Part model, mm, in its own coordinate system. Give positions to 0.01 mm unless a question says otherwise; leave off trailing zeros. Loops run counter-clockwise (first coordinate to the right, second up) from the corner with the lowest first, then second, coordinate; pieces in that order, holes last. Notation, with made-up numbers: (6, 71.5) -> (11, 71.5) arc R21 cw to (11, 93.5) -> close; hole circle Ø3 at (19, 34.25). An arc over 180 degrees is marked (long way). Write item = value, one per line.
from build123d import *

# Parameters (mm, degrees)
CYLINDER_R        = 0.34
CYLINDER_DEPTH    = 12.5
CYLINDER002_R     = 0.24
CYLINDER002_DEPTH = 2.65


with BuildPart() as cone:
    # Cone → Cone (revolve)
    with BuildSketch(Plane(origin=(0, 0, -3.55), x_dir=(1, 0, 0), z_dir=(0, -1, 0))):
        Polygon((0, 0), (0.24, 0.9), (0, 0.9), align=None)
    revolve(axis=Axis((0, 0, -3.55), (0, 0, 1)))


with BuildPart() as body:
    # Cylinder → Cylinder (new body)
    with BuildSketch(Plane.XY):
        Circle(CYLINDER_R)
    extrude(amount=CYLINDER_DEPTH)


with BuildPart() as pin:
    # Cylinder002 → Cylinder002 (new body)
    with BuildSketch(Plane.XY.offset(-2.65)):
        Circle(CYLINDER002_R)
    extrude(amount=CYLINDER002_DEPTH)


with BuildPart() as pogo_pin:
    # Sphere → Sphere (revolve)
    with BuildSketch(Plane(origin=(0, 0, 12.5), x_dir=(1, 0, 0), z_dir=(0, -1, 0))):
        with BuildLine():
            ThreePointArc((0.34, 0), (0.240416, 0.240416), (0, 0.34))
            Line((0, 0.34), (0, 0))
            Line((0, 0), (0.34, 0))
        make_face()
    revolve(axis=Axis((0, 0, 12.5), (0, 0, 1)))

    # Fusion001: union Cone, Body, Pin
    add(cone.part)
    add(body.part)
    add(pin.part)


solid = pogo_pin.part
1) Slice it at A-A, the plane z = -0.75. List the corners of the cut face in (x, y).
Resolved:
outline = circle Ø0.48 at (0, 0)
2) Slice it at B-B, the plane z = 4.5. List the corners of the cut face in (x, y), and give its area (3 significant figures).
Resolved:
outline = circle Ø0.68 at (0, 0)
area = 0.363 mm²
3) Drill centre lines: line 1 along Y through (x, z) = (0, -1.25); line 2 along Y through (x, z) = (-0.05, 12.25); line 3 along X through (y, z) = (0.1, 2.75). Where is each one in solid material? Low to high. Write a range as [from, to].
Resolved:
line_1 = [-0.24, 0.24]
line_2 = [-0.34, 0.34]
line_3 = [-0.32, 0.32]
